Here's how the part is built. I have some questions about the finished solid (model axes, mm). A direction names the side the tool comes from. Coordinates: 2 decimals unless noted, no trailing zeros. Write each loop counter-clockwise with the first axis right and the second up, starting at its lowest first coordinate (ties: lowest second). Pieces come first, ordered by that corner, then holes. Notation, with made-up numbers: (-29.75, -6) -> (20.25, -6) arc R34 cw to (20.25, 30) -> close; hole circle Ø11 at (5, 20). An arc over 180 degrees is marked (long way). Put each result on its own line as item: value.
```python
from build123d import *

# Parameters (mm, degrees)
F0_R     = 31.75
F1_DEPTH = 12.7
F2_W     = 57.15
F2_H     = 19.05
F3_DEPTH = 12.7
F4_T     = -5.715
F5_R     = 3.81
F6_DEPTH = 41.276


with BuildPart() as f1:
    # F0 (on Top) → F1 (new body)
    with BuildSketch(Plane.XY):
        Circle(F0_R)
    extrude(amount=F1_DEPTH)

    # F2 (on Top) → F3 (join)
    with BuildSketch(Plane.XY):
        Rectangle(F2_W, F2_H)
    extrude(amount=-F3_DEPTH)

    # F4
    f4_openings = [f1.faces().sort_by_distance(p)[0] for p in [
        (0, 0, -12.7),
    ]]
    offset(amount=F4_T, openings=f4_openings, kind=Kind.INTERSECTION)

    # F5 (on face) → F6 (cut, through all)
    with BuildSketch(Plane.XZ.offset(9.525)):
        with Locations((0, -6.35)):
            Circle(F5_R)
    extrude(amount=-F6_DEPTH, mode=Mode.SUBTRACT)


solid = f1.part
```
Item 1: Imagine slicing it at B-B on z = -6.35. Write out the boundary of the cut face in (x, y) (3 decimals).
Output:
outline: (-28.575, -9.525) -> (-3.81, -9.525) -> (-3.81, -3.81) -> (-22.86, -3.81) -> (-22.86, 3.81) -> (-3.81, 3.81) -> (-3.81, 9.525) -> (-28.575, 9.525) -> close; (3.81, -9.525) -> (28.575, -9.525) -> (28.575, 9.525) -> (3.81, 9.525) -> (3.81, 3.81) -> (22.86, 3.81) -> (22.86, -3.81) -> (3.81, -3.81) -> close
Item 2: If we mould it in two halves opening along Y, with no side actions, what happens to faces 1 (the flat face through (-0.4, -9.525, -10.5)), 2 (the flat face through (0, 3.81, -1)), 3 (the cylindrical face through (-0.83, 6.63, -10.07))? For each: released by +Y, released by -Y, zero draft, split by the parting line, or undercut.
Output:
face 1: released by -Y
face 2: undercut
face 3: zero draft
Item 3: Imagine slicing it at D-D on y = 11. Write out the boundary of the cut face in (x, z) (3 decimals).
Output:
outline: (-29.784, 0) -> (29.784, 0) -> (29.784, 12.7) -> (-29.784, 12.7) -> close; hole (-23.597, 5.715) -> (23.597, 5.715) -> (23.597, 6.985) -> (-23.597, 6.985) -> close
Item 4: Which directions (+Z, -Z, +X, -X, +Y, -Y) give clear straight access to the entire face, cutting with the end or side of a thin tool? Please do faces 4 (the flat face through (0, -3.81, -1)), 5 (the flat face through (-28.575, 0, -6)), 6 (the flat face through (-0.4, 9.525, -10.5)), 7 (the flat face through (0, -5, 5.715)).
Output:
face 4: -Z
face 5: -Z, -X, +Y, -Y
face 6: -Z, +X, -X, +Y
face 7: none
Item 5: Imagine slicing it at C-C on y = 0. Write out the boundary of the cut face in (x, z) (3 decimals).
Output:
outline: (-31.75, 0) -> (-28.575, 0) -> (-28.575, -12.7) -> (-22.86, -12.7) -> (-22.86, 5.715) -> (-26.035, 5.715) -> (-26.035, 6.985) -> (26.035, 6.985) -> (26.035, 5.715) -> (22.86, 5.715) -> (22.86, -12.7) -> (28.575, -12.7) -> (28.575, 0) -> (31.75, 0) -> (31.75, 12.7) -> (-31.75, 12.7) -> close
Item 6: For P1, Ø5, axis at y = -18, z = 1.5, coming from the +X side; P2, Ø10, axis at x = 0, z = -6.35, coming from the +Y side (3 decimals); P3, Ø1.5, axis at x = -14, z = -3.5, coming from the -Y side (3 decimals); P4, Ø6, axis at x = 0, z = -6.35, coming from the -Y side, each with a flat end and sliding along its axis, tell me the tip position at first contact or that it passes through.
Output:
P1: stops at x = 27.71
P2: stops at y = 9.525
P3: stops at y = -9.525
P4: passes through
Item 7: Please list where these lines run through material, in increasing order: line 1 along Z through (x, y) = (0, -6.3) (3 decimals); line 2 along Y through (x, z) = (0, 6.6) (3 decimals); line 3 along Z through (x, y) = (-18, -14.5) (3 decimals). Write a range as from..to.
Output:
line 1: z = -12.7..-10.16, -2.54..5.715, 6.985..12.7
line 2: y = -31.75..-26.035, 26.035..31.75
line 3: z = 0..5.715, 6.985..12.7
Item 8: Imagine slicing it at A-A on x = 0. Write out the boundary of the cut face in (y, z) (3 decimals).
Output:
outline: (-31.75, 0) -> (-9.525, 0) -> (-9.525, -2.54) -> (-3.81, -2.54) -> (-3.81, 5.715) -> (-26.035, 5.715) -> (-26.035, 6.985) -> (26.035, 6.985) -> (26.035, 5.715) -> (3.81, 5.715) -> (3.81, -2.54) -> (9.525, -2.54) -> (9.525, 0) -> (31.75, 0) -> (31.75, 12.7) -> (-31.75, 12.7) -> close; (-9.525, -12.7) -> (-3.81, -12.7) -> (-3.81, -10.16) -> (-9.525, -10.16) -> close; (3.81, -12.7) -> (9.525, -12.7) -> (9.525, -10.16) -> (3.81, -10.16) -> close
